```python
from build123d import *

# Parameters (mm, degrees)
F0_W      = 50
F0_H      = 30
F1_DEPTH  = 3
F2_SIZE   = 3
F4_R      = 2.5
F4_R_2    = 2
F4_R_3    = 3
F5_DEPTH  = 6
F6_D      = 2
F6_DEPTH  = 7
F6_TIP    = 0.600860619
F7_D      = 1.75
F7_DEPTH  = 7
F7_TIP    = 0.5257530416
F8_D      = 1.5
F8_DEPTH  = 7
F8_TIP    = 0.4506454643
F9_D      = 1.25
F9_DEPTH  = 7
F9_TIP    = 0.3755378869
F10_D     = 2.25
F10_DEPTH = 7
F10_TIP   = 0.6759681964
F11_D     = 2.5
F11_DEPTH = 7
F11_TIP   = 0.7510757738
F12_D     = 3
F12_DEPTH = 7
F12_TIP   = 0.9012909285


with BuildPart() as f1:
    # F0 (on Top) → F1 (new body)
    with BuildSketch(Plane.XY):
        Rectangle(F0_W, F0_H)
    extrude(amount=-F1_DEPTH)

    # F2
    f2_edges = [f1.edges().sort_by_distance(p)[0] for p in [
        (-25, -15, -1.5),
        (25, -15, -1.5),
        (25, 15, -1.5),
        (-25, 15, -1.5),
    ]]
    chamfer(f2_edges, length=F2_SIZE)

    # F4 (on offset) → F5 (join)
    with BuildSketch(Plane.XY.offset(6)):
        with Locations((-20, 0)):
            Circle(F4_R)
        with Locations((-10, 0)):
            Circle(F4_R)
        Circle(F4_R)
        with Locations((10, 0)):
            Circle(F4_R)
        with Locations((20, 0)):
            Circle(F4_R)
        with Locations((-20, 10)):
            Circle(F4_R_2)
        with Locations((-10, 10)):
            Circle(F4_R_2)
        with Locations((0, 10)):
            Circle(F4_R_2)
        with Locations((10, 10)):
            Circle(F4_R_2)
        with Locations((20, 10)):
            Circle(F4_R_2)
        with Locations((-20, -10)):
            Circle(F4_R_3)
        with Locations((-10, -10)):
            Circle(F4_R_3)
        with Locations((0, -10)):
            Circle(F4_R_3)
        with Locations((10, -10)):
            Circle(F4_R_3)
        with Locations((20, -10)):
            Circle(F4_R_3)
    extrude(amount=-F5_DEPTH)

    # F6
    with Locations(Plane.XY.offset(6)):
        with Locations((0, 0), (10, 10), (-10, -10)):
            Hole(F6_D / 2, depth=F6_DEPTH)
            with Locations((0, 0, -(F6_DEPTH + F6_TIP / 2))):  # 118° drill point
                Cone(0, F6_D / 2, F6_TIP, mode=Mode.SUBTRACT)

    # F7
    with Locations(Plane.XY.offset(6)):
        with Locations((-20, -10), (-10, 0), (0, 10)):
            Hole(F7_D / 2, depth=F7_DEPTH)
            with Locations((0, 0, -(F7_DEPTH + F7_TIP / 2))):  # 118° drill point
                Cone(0, F7_D / 2, F7_TIP, mode=Mode.SUBTRACT)

    # F8
    with Locations(Plane.XY.offset(6)):
        with Locations((-20, 0), (-10, 10)):
            Hole(F8_D / 2, depth=F8_DEPTH)
            with Locations((0, 0, -(F8_DEPTH + F8_TIP / 2))):  # 118° drill point
                Cone(0, F8_D / 2, F8_TIP, mode=Mode.SUBTRACT)

    # F9
    with Locations(Plane.XY.offset(6)):
        with Locations((-20, 10)):
            Hole(F9_D / 2, depth=F9_DEPTH)
            with Locations((0, 0, -(F9_DEPTH + F9_TIP / 2))):  # 118° drill point
                Cone(0, F9_D / 2, F9_TIP, mode=Mode.SUBTRACT)

    # F10
    with Locations(Plane.XY.offset(6)):
        with Locations((0, -10), (10, 0), (20, 10)):
            Hole(F10_D / 2, depth=F10_DEPTH)
            with Locations((0, 0, -(F10_DEPTH + F10_TIP / 2))):  # 118° drill point
                Cone(0, F10_D / 2, F10_TIP, mode=Mode.SUBTRACT)

    # F11
    with Locations(Plane.XY.offset(6)):
        with Locations((10, -10), (20, 0)):
            Hole(F11_D / 2, depth=F11_DEPTH)
            with Locations((0, 0, -(F11_DEPTH + F11_TIP / 2))):  # 118° drill point
                Cone(0, F11_D / 2, F11_TIP, mode=Mode.SUBTRACT)

    # F12
    with Locations(Plane.XY.offset(6)):
        with Locations((20, -10)):
            Hole(F12_D / 2, depth=F12_DEPTH)
            with Locations((0, 0, -(F12_DEPTH + F12_TIP / 2))):  # 118° drill point
                Cone(0, F12_D / 2, F12_TIP, mode=Mode.SUBTRACT)


solid = f1.part
```
CAD build for the part. Positions are in the model's coordinates, mm. A direction names the side the tool comes from. Coordinates: 2 decimals unless noted, no trailing zeros. Write each loop counter-clockwise with the first axis right and the second up, starting at its lowest first coordinate (ties: lowest second). Pieces come first, ordered by that corner, then holes. Notation, with made-up numbers: (48, 77.25) -> (55, 77.25) arc R24 ccw to (55, 108.25) -> close; hole circle Ø10 at (68, 80). An arc over 180 degrees is marked (long way). Use CSV: the item, a comma, the result in double quotes. Start each with the question number.
Item 1: Drop flat-ended pins along their axis: P1, Ø1.1, axis at x = -20, y = 10, coming from the +Z side; P2, Ø4, axis at y = -6.5, z = 3, coming from the +X side; P3, Ø1.2, axis at x = -20, y = 0, coming from the +Z side. Give the stop position or say it passes through.
Item 2: Band-saw the part on C-C, the plane x = 15.5. Write the cut outline in (y, z), plus the area to 3 significant figures.
Item 3: Band-saw the part on B-B, the plane y = 2. Write the cut outline in (x, z), plus the area to 3 significant figures.
Item 4: Band-saw the part on A-A, the plane z = 4.75. Give the number of separate pieces and of enclosed holes in the cut face, plus the area to 3 significant figures.
Item 5: Band-saw the part on D-D, the plane y = 5.25. Write the cut outline in (x, z).
Item 6: Wall check: probe 1 along Y at (x, z) = (-10, 2) (3 decimals); probe 2 along Y at (x, z) = (-20, 1.5) (3 decimals); probe 3 along X at (y, z) = (-2.25, 5.25). Give the ranges that are in metal, low to high.
Item 7: Two-plate mould, pull along Y, no slides. Class faces 3 (the flat face through (25, 0, -1)), 4 (the cylindrical face through (-9.45, 10.51, 2.45)), 5 (the flat face through (23, 14, -1)), 6 (the conical face through (-10.138, -10.106, -1.497)): +Y half, -Y half, draft (parallel to the pull), parting line (faces both ways), or undercut.
Item 8: Tool access for faces 1 (the cylindrical face through (-9.126, 0.038, 2.451)), 2 (the flat face through (-19, -11, 6)): list every direction of +Z, -Z, +X, -X, +Y, -Y with a clear straight run to the whole face (end or side of a thin tool).
Response values:
1,P1,"stops at z = -1.05"
1,P2,"stops at x = 22.6"
1,P3,"stops at z = -1.09"
2,outline,"(-15, -3) -> (15, -3) -> (15, 0) -> (-15, 0) -> close"
2,area,"90.0 mm2"
3,outline,"(-25, -3) -> (25, -3) -> (25, 0) -> (21.5, 0) -> (21.5, 6) -> (18.5, 6) -> (18.5, 0) -> (11.5, 0) -> (11.5, 6) -> (8.5, 6) -> (8.5, 0) -> (1.5, 0) -> (1.5, 6) -> (-1.5, 6) -> (-1.5, 0) -> (-8.5, 0) -> (-8.5, 6) -> (-11.5, 6) -> (-11.5, 0) -> (-18.5, 0) -> (-18.5, 6) -> (-21.5, 6) -> (-21.5, 0) -> (-25, 0) -> close"
3,area,"240 mm2"
4,separate pieces,"15"
4,enclosed holes,"15"
4,area,"252 mm2"
5,outline,"(-25, -3) -> (25, -3) -> (25, 0) -> (-25, 0) -> close"
6,probe 1,"y = -13 to -11, -9 to -7, -2.5 to -0.875, 0.875 to 2.5, 8 to 9.25, 10.75 to 12"
6,probe 2,"y = -13 to -10.875, -9.125 to -7, -2.5 to -0.75, 0.75 to 2.5, 8 to 9.375, 10.625 to 12"
6,probe 3,"x = -21.09 to -18.91, -11.09 to -8.91, -1.09 to 1.09, 8.91 to 11.09, 18.91 to 21.09"
7,face 3,"draft"
7,face 4,"undercut"
7,face 5,"+Y half"
7,face 6,"undercut"
8,face 1,"+Z"
8,face 2,"+Z, +X, -X, +Y, -Y"
